Design review of the part built by this model. Coordinates are the model's own, in mm. A direction names the side the tool comes from. Give positions to 0.01 mm unless a question says otherwise; leave off trailing zeros. Order: outer loops, then holes, each group sorted by start corner. A loop starts at its lowest first (then second) coordinate and runs counter-clockwise, first axis right, second up. Notation, with made-up numbers: (33.5, 69.25) -> (64.5, 69.25) arc R12 ccw to (64.5, 83.25) -> close; hole circle Ø10 at (43.5, 89.25). An arc over 180 degrees is marked (long way). One line per item, written item: value. Start each with the question number.
1) Consider section A-A (x = 1.75). State the section outline as (y, z) points.
2) The part is to be moulded in two halves that separate along Y. For faces 3 (the face through (0, 0, 0)), 4 (the face through (3.137, 1.987, -0.626)), 5 (the face through (5.18, 0.49, 0.86)), say which applies: released by +Y, released by -Y, zero draft, split by the parting line, or undercut.
3) Wall thickness on line 1 along Y through (x, z) = (5.25, 0.5); line 2 along Z through (x, y) = (4.25, 0.45); line 3 along Z through (x, y) = (5, 0.05): over which ranges is each line inside the solid? List them lowest first. Write a range as from..to.
4) For pin 1 (1.5 mm diameter, centred on y = 1, z = 0.5, fed in from -X), flat-tipped, find the tip position at first contact; note if it passes through.
5) Tool access review of faces 1 (the face through (6.35, -1, 1)), 2 (the face through (5.18, -0.49, -0.86)): name each direction out of +Z, -Z, +X, -X, +Y, -Y from which nothing blocks a thin tool from reaching the whole face with its end or side.
Autodesk Inventor part; units mm, degrees
ref_plane "Work Plane1" through (3.175, 0, 0) normal (0, 0.5, 0.866) x (1, 0, 0)
ref_plane "YZ Plane" through (0, 0, 0) normal (1, 0, 0) x (0, 1, 0)
ref_plane "XZ Plane" through (0, 0, 0) normal (0, 1, 0) x (-1, 0, 0)
sketch "Sketch1" plane through (0, 0, 0) normal (0, 0, 1) x (1, 0, 0)
  line L0 (0, 0) -> (3.4036, 0)
  line L1 (6.35, 1.1438) -> (6.35, 2.0828)
  line L2 (6.35, 2.0828) -> (0, 2.0828)
  line L3 (6.35, 1.1438) -> (4.064, 1.1438)
  line L4 (4.064, 1.1438) -> (3.4036, 0)
  line L5 (0, -0.4166) -> (0, 2.4994)
  line L6 (0, 2.0828) -> (0, 0)
  dimension "d0" = 2.286
  dimension "d1" = 60
  dimension "d2" = 4.1656
  dimension "d3" = 2.2877
  dimension "d5" = 6.35
revolve "Body" add sketch "Sketch1" angle 360 about axis through (0, 0, 0) along (1, 0, 0)
chamfer "Chamfer1" distance 0.4869 angle 45 1 edges at (6.35, -2.0828, 0) measured on face at (6.35, 1.7386, -0.2574)
sketch "Sketch2" plane through (6.35, 0, 0) normal (1, 0, 0) x (0, 0, -1)
  circle A0 centre (0, 0) radius 1.1438
  line L0 (-0.5719, 0.9906) -> (0.5719, 0.9906)
  line L1 (0.5719, 0.9906) -> (1.1438, 0)
  line L2 (1.1438, 0) -> (0.5719, -0.9906)
  line L3 (0.5719, -0.9906) -> (-0.5719, -0.9906)
  line L4 (-0.5719, -0.9906) -> (-1.1438, 0)
  line L5 (-1.1438, 0) -> (-0.5719, 0.9906)
  point P0 (0, 0)
  point P1 (0, 0)
extrude "Slot" add sketch "Sketch2" against normal up to next contours L1 A0 | A0 L2 | L0 A0 | A0 L3 | L5 A0 | A0 L4
thread "Thread"
chamfer "Chamfer2" distance 0.4869 angle 45 1 edges at (0, -2.0828, 0) measured on face at (1.9544, 2.076, -0.1676)
ref_plane "Work Plane1" through (3.175, 0, 0) normal (0, 0.5, 0.866) x (1, 0, 0)
equation "\"d0\" = INTI"
equation "\"d2\" = NND"
equation "\"d3\" = 1.1547 * SW"
equation "\"d5\" = NLG"
equation "\"d7\" = -0.5 * GD1 + 0.5 * NND"
equation "\"d8\" = FAWI"
equation "\"d29\" = -0.5 * GD1 + 0.5 * NND"
equation "\"d11\" = NLG"
equation "\"d13\" = -0.5 * GD1 + 0.5 * NND"
equation "\"d14\" = FAWI"
equation "\"d30\" = -0.5 * GD1 + 0.5 * NND"
equation "\"NND\" = 4.1656"
equation "\"NLG\" = 6.35"
equation "\"INTI\" = 2.286"
equation "\"FAWI\" = 45deg"
equation "\"SW\" = 1.9812"
equation "\"GD1\" = 3.19177"
equation "\"FAWI1\" = 45deg"
equation "\"SPD\" = 2.2098"
equation "\"SEWI\" = 90deg"
equation "\"TOA\" = 30deg"
equation "\"ZLG\" = 1.0922"
equation "\"ZD\" = 2.7686"
equation "\"HHPTC\" = 0.79375"
equation "\"THREADDIA\" = 4.1656"
equation "\"OPR\" = 3.1242"
equation "\"E0\" = 1.155 * SW"
properties part number "ANSI B18.3 - 8-32 UNC x 0.25" material "Steel, Mild"
Checked values:
1. outline: circle Ø4.17 at (0, 0)
2. face 3: zero draft
2. face 4: split by the parting line
2. face 5: undercut
3. line 1: y = -2.02..-0.99, 0.99..2.02
3. line 2: z = -2.03..-0.88, 0.88..2.03
3. line 3: z = -2.08..-1.11, 1.11..2.08
4. pin 1: stops at x = 0
5. face 1: +Z, -Z, +X, +Y, -Y
5. face 2: +X
